Check sheet for the modelled part. Datum: model origin and axes. Units: mm. A direction names the side the tool comes from. Give positions to 0.01 mm unless a question says otherwise; leave off trailing zeros. Order: outer loops, then holes, each group sorted by start corner. A loop starts at its lowest first (then second) coordinate and runs counter-clockwise, first axis right, second up.
Item 1: Material ranges on line 1 along Y through (x, z) = (-29, 129); line 2 along X through (y, z) = (14.5, 62) (3 decimals); line 3 along Y through (x, z) = (-4, 95), recorded low to high.
Item 2: Sectioned sample at B-B on z = 408.5. Record the boundary of the cut face in (x, y) (3 decimals).
Item 3: Release check for a two-part mould opening along Y. For faces 1 (the flat face through (-41, -33.933, 232)), 2 (the flat face through (-40, 42.267, 232)), 3 (the flat face through (-2, 4, 0)), 4 (the flat face through (-40, -30.758, 232)) record: released by +Y, released by -Y, zero draft, split by the parting line, or undercut.
Item 4: Sectioned sample at C-C on y = 26.5. Record the boundary of the cut face in (x, z) (3 decimals).
Item 5: Gauge pin test, flat end, axial feed: P1, Ø2, axis at y = -7, z = 272, coming from the -X side (3 decimals). Record the tip position at first contact, or that the pin passes through.
Item 6: Access from +Z, -Z, +X, -X, +Y, -Y to the whole of each face (thin tool, end or side, straight path). Record for faces 5 (the flat face through (-3.175, 5, 232)), 6 (the flat face through (0, 4, 232)).
Item 7: Sectioned sample at A-A on x = -47.5. Record the boundary of the cut face in (y, z).
from build123d import *

# Parameters (mm, degrees)
F1_DEPTH = 469.9
F2_R     = 5.08


with BuildPart() as f1:
    # F0 (on Top) → F1 (new body)
    with BuildSketch(Plane.XY):
        with BuildLine():
            Line((-5.715, 42.267205), (-76.2, 42.267205))
            Line((-76.2, 42.267205), (-76.2, 39.092205))
            Line((-76.2, 39.092205), (-5.715, 39.092205))
            ThreePointArc((-5.715, 39.092205), (-3.918949, 38.348257), (-3.175, 36.552205))
            Line((-3.175, 36.552205), (-3.175, -28.217795))
            ThreePointArc((-3.175, -28.217795), (-3.918949, -30.013846), (-5.715, -30.757795))
            Line((-5.715, -30.757795), (-76.2, -30.757795))
            Line((-76.2, -30.757795), (-76.2, -33.932795))
            Line((-76.2, -33.932795), (-5.715, -33.932795))
            ThreePointArc((-5.715, -33.932795), (-1.673885, -32.25891), (0, -28.217795))
            Line((0, -28.217795), (0, 36.552205))
            ThreePointArc((0, 36.552205), (-1.673885, 40.593321), (-5.715, 42.267205))
        make_face()
    extrude(amount=F1_DEPTH)

    # F2
    f2_edges = [f1.edges().sort_by_distance(p)[0] for p in [
        (-76.2, -32.345295, 469.9),
        (-76.2, 40.679705, 469.9),
    ]]
    fillet(f2_edges, radius=F2_R)


solid = f1.part
Report:
1. line 1: y = -33.93 to -30.76, 39.09 to 42.27
1. line 2: x = -3.175 to 0
1. line 3: y = -33.67 to -30.09, 38.43 to 42
2. outline: (-76.2, -33.933) - (-5.715, -33.933) arc R5.715 ccw to (0, -28.218) - (0, 36.552) arc R5.715 ccw to (-5.715, 42.267) - (-76.2, 42.267) - (-76.2, 39.092) - (-5.715, 39.092) arc R2.54 cw to (-3.175, 36.552) - (-3.175, -28.218) arc R2.54 cw to (-5.715, -30.758) - (-76.2, -30.758) - close
3. face 1: released by -Y
3. face 2: released by +Y
3. face 3: zero draft
3. face 4: undercut
4. outline: (-3.175, 0) - (0, 0) - (0, 469.9) - (-3.175, 469.9) - close
5. P1: stops at x = -3.175
6. face 5: +Z, -Z, -X
6. face 6: +Z, -Z, +X, +Y, -Y
7. outline: (-33.93, 0) - (-30.76, 0) - (-30.76, 469.9) - (-33.93, 469.9) - close; (39.09, 0) - (42.27, 0) - (42.27, 469.9) - (39.09, 469.9) - close
